from build123d import *

# Parameters (mm, degrees)
BOSS_EXTRUDE2_DEPTH = 3.175
CUT_EXTRUDE1_DEPTH  = 7.35


with BuildPart() as part:
    # Sketch2 → Boss-Extrude2 (new body, symmetric)
    with BuildSketch(Plane(origin=(0, 0, 0), x_dir=(1, 0, 0), z_dir=(0, 1, 0))):
        with BuildLine():
            Line((0, 50.8), (5.699182497, 35.141624781))
            ThreePointArc((5.699182497, 35.141624781), (4.697625818, 30.400196659), (0, 29.21))
            ThreePointArc((0, 29.21), (-40.712457699, 16.982230342), (-43.994090512, -25.4))
            Line((-43.994090512, -25.4), (-33.283131039, -12.635175567))
            ThreePointArc((-33.283131039, -12.635175567), (-28.676155496, -11.131835033), (-25.296602045, -14.605))
            ThreePointArc((-25.296602045, -14.605), (5.64918596, -43.749137789), (43.994090512, -25.4))
            Line((43.994090512, -25.4), (27.583948542, -22.506449213))
            ThreePointArc((27.583948542, -22.506449213), (23.978529677, -19.268361626), (25.296602045, -14.605))
            ThreePointArc((25.296602045, -14.605), (35.063271738, 26.766907447), (0, 50.8))
        make_face()
        Polygon((0, 10.998522628), (9.525, 5.499261314), (9.525, -5.499261314), (0, -10.998522628), (-9.525, -5.499261314), (-9.525, 5.499261314), align=None, mode=Mode.SUBTRACT)
    extrude(amount=BOSS_EXTRUDE2_DEPTH, both=True)

    # Sketch3 → Cut-Extrude1 (cut, through all)
    with BuildSketch(Plane(origin=(0, 3.175, 0), x_dir=(1, 0, 0), z_dir=(0, 1, 0))):
        with BuildLine():
            ThreePointArc((0, 29.21), (-36.786884898, 21.158593478), (-48.137903328, -14.747595795))
            ThreePointArc((-48.137903328, -14.747595795), (-32.049598102, 15.970797155), (0, 29.21))
        make_face()
        with BuildLine():
            ThreePointArc((11.297159061, 49.062445064), (29.855915106, 19.77036756), (25.296602045, -14.605))
            ThreePointArc((25.296602045, -14.605), (36.717321909, 21.279080109), (11.297159061, 49.062445064))
        make_face()
        with BuildLine():
            ThreePointArc((-25.296602045, -14.605), (0.069562989, -42.437673587), (36.840744267, -34.314849269))
            ThreePointArc((36.840744267, -34.314849269), (2.193682996, -35.741164715), (-25.296602045, -14.605))
        make_face()
    extrude(amount=-CUT_EXTRUDE1_DEPTH, mode=Mode.SUBTRACT)


solid = part.part
For this review, take the finished solid that the model builds, in its own axes (mm). A direction names the side the tool comes from. Give positions to 0.01 mm unless a question says otherwise; leave off trailing zeros. Order: outer loops, then holes, each group sorted by start corner. A loop starts at its lowest first (then second) coordinate and runs counter-clockwise, first axis right, second up. Notation, with made-up numbers: M 50.5,26 L 100.5,26 A22 cw 100.5,57 Z; hole C 37,35.5 d4. An arc over 180 degrees is marked long. Answer in a Markdown table with one row per item. Add a question column.
(1) Consider section A-A on x = 3. State the section outline as (y, z) points (3 decimals), and give its area (3 significant figures).
(2) Wall thickness on probe 1 along Z at (x, y) = (-4.5, -2); probe 2 along X at (y, z) = (-2.75, 7.5); probe 3 along Z at (x, y) = (7.5, 1): over which ranges is each line inside the solid? List them lowest first. Write a range as [from, to].
(3) Consider section D-D on x = 16. State the section outline as (y, z) points (3 decimals).
(4) Mouldability with a two-part tool opening along X and no side actions: class faces 4 (the face through (-38.714, 0.044, 19.107)), 5 (the face through (-32.414, 0.044, -15.635)), 6 (the face through (-4.83, 0.04, -8.21)), 7 (the face through (24, 0.04, 19.34)) as +X half, -X half, draft (parallel to the pull), parting line (faces both ways), or undercut.
(5) Consider section B-B on z = 18. State the section outline as (x, y) points (3 decimals).
(6) For faces 1 (the face through (2.81, 0.04, -43.08)), 2 (the face through (35.904, 0.044, 23.973)), 3 (the face through (-4.696, 0.044, 8.287)), list the 3-axis set-ups (+Z, -Z, +X, -X, +Y, -Y) from which the entire face can be reached by the end or side of a thin tool; tool diameter is ignored.
(7) For pin 1 (3 mm diameter, centred on x = 18.5, y = 1, fed in from -Z); pin 2 (1 mm diameter, centred on y = -1.5, z = 7.5, fed in from -X), all flat-tipped, find the tip position at first contact; note any pin that passes through.
(8) Consider section C-C on y = 1.25. State the section outline as (x, z) points (3 decimals), and give its area (3 significant figures).
Evaluation:
| question | item | result |
|---|---|---|
| 1 | outline | M -3.175,-50.68 L 3.175,-50.68 L 3.175,-42.558 L -3.175,-42.558 Z; M -3.175,-29.284 L 3.175,-29.284 L 3.175,-9.266 L -3.175,-9.266 Z; M -3.175,9.266 L 3.175,9.266 L 3.175,35.99 L -3.175,35.99 Z |
| 1 | area | 348 mm^2 |
| 2 | probe 1 | z = [-28.81, -8.4], [8.4, 33.08] |
| 2 | probe 2 | x = [-46.62, -6.06], [6.06, 28.33] |
| 2 | probe 3 | z = [-50.04, -6.67], [6.67, 37.11] |
| 3 | outline | M -3.175,-44.943 L 3.175,-44.943 L 3.175,38.095 L -3.175,38.095 Z |
| 4 | face 4 | undercut |
| 4 | face 5 | -X half |
| 4 | face 6 | undercut |
| 4 | face 7 | +X half |
| 5 | outline | M -47.262,-3.175 L -37.785,-3.175 L -37.785,3.175 L -47.262,3.175 Z; M -22.935,-3.175 L 23.798,-3.175 L 23.798,3.175 L -22.935,3.175 Z |
| 6 | face 1 | -X, +Y, -Y |
| 6 | face 2 | +X, +Y, -Y |
| 6 | face 3 | +Y, -Y |
| 7 | pin 1 | stops at z = -43.92 |
| 7 | pin 2 | stops at x = -46.76 |
| 8 | outline | M -48.138,14.748 A50.8 ccw 0,-29.21 A4.582 cw 5.699,-35.142 L 0,-50.8 A37.594 ccw 11.297,-49.062 A50.8 ccw 25.297,14.605 A4.582 cw 27.584,22.506 L 43.994,25.4 A37.594 ccw 36.841,34.315 A50.8 ccw -25.297,14.605 A4.582 cw -33.283,12.635 L -43.994,25.4 A37.594 ccw Z; hole M -9.525,-5.499 L 0,-10.999 L 9.525,-5.499 L 9.525,5.499 L 0,10.999 L -9.525,5.499 Z |
| 8 | area | 4,020 mm^2 |
